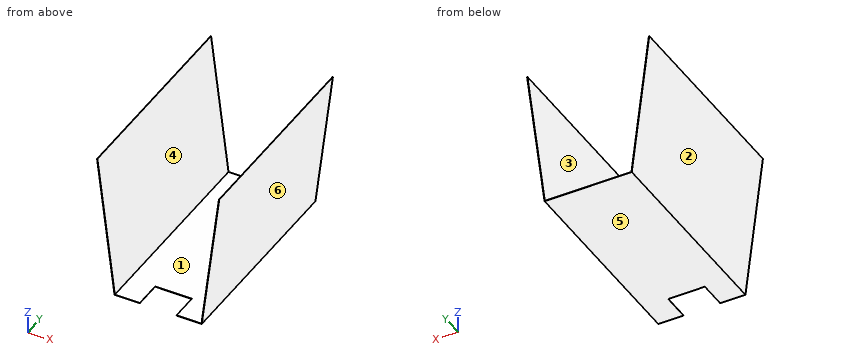
```python
from build123d import *

# Parameters (mm, degrees)
F1_DEPTH      = 565.15
F2_T          = -0.762
F3_W          = 101.6
F3_H          = 76.2
F4_DEPTH      = 81.28
F4_DEPTH_BACK = 106.68


with BuildPart() as f1:
    # F0 (on Front) → F1 (new body)
    with BuildSketch(Plane.XZ):
        Polygon((-120.65, 0), (0, 0), (120.65, 0), (169.0323730705, 394.0428072939), (-169.0323730705, 394.0428072939), align=None)
    extrude(amount=-F1_DEPTH)

    # F2
    f2_openings = [f1.faces().sort_by_distance(p)[0] for p in [
        (0, 0, 207.990156),
        (0, 282.575, 394.042807),
        (0, 565.15, 207.990156),
    ]]
    offset(amount=F2_T, openings=f2_openings)

    # F3 (on Top) → F4 (cut, two sides)
    with BuildSketch(Plane.XY) as f4_sk:
        with Locations((0, 38.1)):
            Rectangle(F3_W, F3_H)
    extrude(amount=-F4_DEPTH, mode=Mode.SUBTRACT)
    extrude(f4_sk.sketch, amount=F4_DEPTH_BACK, mode=Mode.SUBTRACT)


solid = f1.part
```
Design review of the part built by this model. Coordinates are the model's own, in mm. Face numbers are marked on the shaded views. A direction names the side the tool comes from. Round coordinates to 2 decimals unless told otherwise and drop trailing zeros. Order: outer loops, then holes, each group sorted by start corner. A loop starts at its lowest first (then second) coordinate and runs counter-clockwise, first axis right, second up. Notation, with made-up numbers: M 40.25,17.25 L 74.25,17.25 A11 ccw 74.25,23.25 Z; hole C 21,-4 d7. An arc over 180 degrees is marked long. Put each result on its own line as item: value.
Q1. Consider section D-D (x = 93). State the section outline as (y, z) points, and give its area (3 significant figures).
Reported:
outline: M 0,0 L 565.15,0 L 565.15,0.76 L 0,0.76 Z
area: 431 mm²
Q2. Draft analysis for pull direction X (two halves, no side actions). For the marked faces 3, 4, 5 and 6, state which applies: released by +X, released by -X, zero draft, split by the parting line, or undercut.
Reported:
face 3: undercut
face 4: undercut
face 5: zero draft
face 6: released by +X
Q3. Consider section C-C (y = 287.5). State the section outline as (x, z) points.
Reported:
outline: M -169.03,394.04 L -120.65,0 L 120.65,0 L 169.03,394.04 L 168.26,394.04 L 119.98,0.76 L -119.98,0.76 L -168.26,394.04 Z
Q4. Insertion check: pin 1 Ø0.8 at (y, z) = (57, 0.5) entering from +X; pin 2 Ø12 at (y, z) = (130.5, 44.5) entering from +X; pin 3 Ø1.5 at (x, y) = (1.5, 207.5) entering from +Z. Each pin has a flat end and moves straight along its axis. Give the tip position at first contact, or say it passes through.
Reported:
pin 1: x = 120.76
pin 2: x = 126.85
pin 3: z = 0.76
Q5. Consider section B-B (z = 52.5). State the section outline as (x, y) points.
Reported:
outline: M -127.1,0 L -126.33,0 L -126.33,565.15 L -127.1,565.15 Z; M 126.33,0 L 127.1,0 L 127.1,565.15 L 126.33,565.15 Z
Q6. To check wall thickness, follow line 1 (Z direction, x = 89, y = 515.5); line 2 (X direction, y = 263.5, z = 167.5); line 3 (X direction, y = 202.5, z = 225). State the ranges of each line that lie inside material, in increasing order.
Reported:
line 1: 0 to 0.76
line 2: -141.22 to -140.45, 140.45 to 141.22
line 3: -148.28 to -147.51, 147.51 to 148.28
Q7. Machinability: for the marked faces 1 and 2, which of the approach directions +Z, -Z, +X, -X, +Y, -Y give a long, thin tool a straight path to every point of the face, cutting with its end or side? Answer none if there is none.
Reported:
face 1: +Z, +Y, -Y
face 2: -Z, -X, +Y, -Y
Q8. Consider section A-A (y = 37). State the section outline as (x, z) points, and give its area (3 significant figures).
Reported:
outline: M -169.03,394.04 L -120.65,0 L -50.8,0 L -50.8,0.76 L -119.98,0.76 L -168.26,394.04 Z; M 50.8,0 L 120.65,0 L 169.03,394.04 L 168.26,394.04 L 119.98,0.76 L 50.8,0.76 Z
area: 710 mm²
